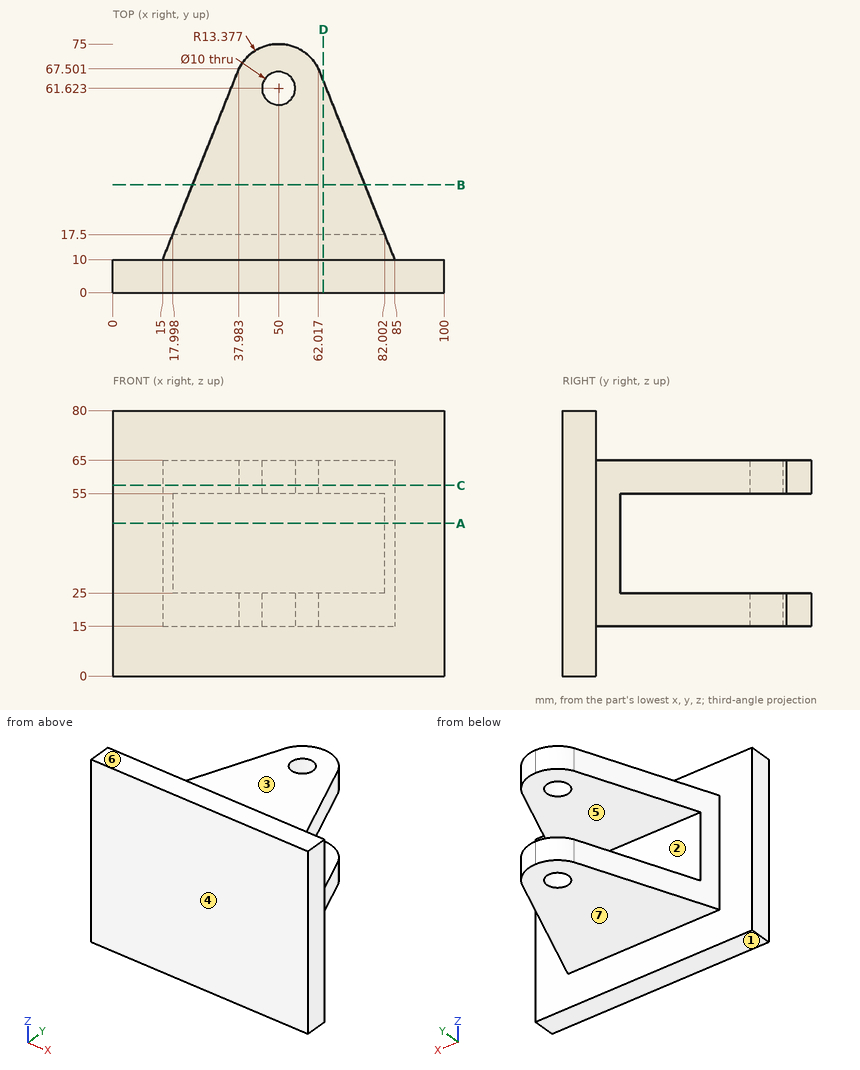
Input: dimensioned drawing with shaded views. Units: mm. Origin: part minimum x, y, z. A direction names the side the tool comes from. Coordinates: 2 decimals unless noted, no trailing zeros. Loops run counter-clockwise (first coordinate to the right, second up) from the corner with the lowest first, then second, coordinate; pieces in that order, holes last.
Q1. Mould query, pull axis Z, two halves, no side actions, for the marked faces 4, 5, 6 and 7. Classes: +Z half, -Z half, draft (parallel to the pull), parting line (faces both ways), or undercut.
Results are:
face 4: draft
face 5: undercut
face 6: +Z half
face 7: -Z half
Q2. Set-up query: the marked faces 1, 2 and 3. Return all of +Z, -Z, +X, -X, +Y, -Y with unobstructed straight access to the full face (end or side cutting, diameter ignored); none if empty.
Results are:
face 1: -Z, +X, -X, +Y, -Y
face 2: +X, -X, +Y
face 3: +Z, +X, -X, +Y
Q3. Section B-B, the plane y = 32.5. Return the cut outline in (x, z).
Results are:
outline: (23.99, 15) - (76.01, 15) - (76.01, 25) - (23.99, 25) - close; (23.99, 55) - (76.01, 55) - (76.01, 65) - (23.99, 65) - close
Q4. Section D-D, the plane x = 63.5. Return the cut outline in (y, z), and give its area (3 significant figures).
Results are:
outline: (0, 0) - (10, 0) - (10, 15) - (63.79, 15) - (63.79, 25) - (17.5, 25) - (17.5, 55) - (63.79, 55) - (63.79, 65) - (10, 65) - (10, 80) - (0, 80) - close
area: 2,100 mm2
Q5. Section C-C, the plane z = 57.5. Return the cut outline in (x, y) (1 decimal).
Results are:
outline: (0, 0) - (100, 0) - (100, 10) - (85, 10) - (62, 67.5) arc R13.4 ccw to (38, 67.5) - (15, 10) - (0, 10) - close; hole circle Ø10 at (50, 61.6)
Q6. Contact query for flat-ended pins moving along their axis: pin 1 (5 mm diameter, centred on y = 14, z = 37, fed in from -X); pin 2 (9 mm diameter, centred on x = 58, z = 37.5, fed in from +Y); pin 3 (6 mm diameter, centred on x = 50, y = 61.62, fed in from +Z); pin 4 (8 mm diameter, centred on x = 56, y = 59, fed in from -Z). Output: stop coordinate, or through.
Results are:
pin 1: stops at x = 15.6
pin 2: stops at y = 17.5
pin 3: passes through
pin 4: stops at z = 15
Q7. Line query: line 1 along Y through (x, z) = (50, 60.25); line 2 along Z through (x, y) = (33.5, 34); line 3 along Y through (x, z) = (35.5, 35). Output: solid intervals per line, ascending.
Results are:
line 1: y = 0 to 56.62, 66.62 to 75
line 2: z = 15 to 25, 55 to 65
line 3: y = 0 to 17.5
Q8. Section A-A, the plane z = 46. Return the cut outline in (x, y).
Results are:
outline: (0, 0) - (100, 0) - (100, 10) - (85, 10) - (82, 17.5) - (18, 17.5) - (15, 10) - (0, 10) - close
